```python
from build123d import *

# Parameters (mm, degrees)
BOSS_EXTRUDE1_DEPTH = 30
SKETCH2_W           = 20
SKETCH2_H           = 8
BOSS_EXTRUDE2_DEPTH = 30
BOSS_EXTRUDE3_DEPTH = 30
FILLET2_R           = 35
FILLET3_R           = 3
SKETCH5_R           = 2.778125
CUT_EXTRUDE2_DEPTH  = 9
SKETCH6_R           = 24.13
BOSS_EXTRUDE4_DEPTH = 30
FILLET4_R           = 40
FILLET5_R           = 10
FILLET6_R           = 2


with BuildPart() as part:
    # Sketch1 → Boss-Extrude1 (new body)
    with BuildSketch(Plane.XY):
        with BuildLine():
            ThreePointArc((66.675, 0), (0, 66.675), (-66.675, 0))
            Line((-66.675, 0), (-57.15, 0))
            ThreePointArc((-57.15, 0), (0, 57.15), (57.15, 0))
            Line((57.15, 0), (66.675, 0))
        make_face()
    extrude(amount=BOSS_EXTRUDE1_DEPTH)

    # Sketch2 → Boss-Extrude2 (add)
    with BuildSketch(Plane.XY.offset(30)):
        with Locations((-71.9125, 4)):
            Rectangle(SKETCH2_W, SKETCH2_H)
        with Locations((71.9125, 4)):
            Rectangle(SKETCH2_W, SKETCH2_H)
    extrude(amount=-BOSS_EXTRUDE2_DEPTH)

    # Sketch4 → Boss-Extrude3 (add)
    with BuildSketch(Plane.XY.offset(30)):
        with BuildLine():
            Line((-89.9125, 40), (-89.9125, 35))
            Line((-89.9125, 35), (-81.9125, 35))
            Line((-81.9125, 35), (-56.749939427, 35))
            ThreePointArc((-56.749939427, 35), (-55.103585117, 37.538653841), (-53.343749634, 40))
            Line((-53.343749634, 40), (-89.9125, 40))
        make_face()
        Polygon((-89.9125, 0), (-81.9125, 0), (-81.9125, 8), (-81.9125, 35), (-89.9125, 35), align=None)
        with BuildLine():
            Line((89.9125, 40), (53.343749634, 40))
            ThreePointArc((53.343749634, 40), (55.103585117, 37.538653841), (56.749939427, 35))
            Line((56.749939427, 35), (81.9125, 35))
            Line((81.9125, 35), (89.9125, 35))
            Line((89.9125, 35), (89.9125, 40))
        make_face()
        Polygon((89.9125, 0), (89.9125, 35), (81.9125, 35), (81.9125, 8), (81.9125, 0), align=None)
    extrude(amount=-BOSS_EXTRUDE3_DEPTH)

    # Fillet2
    fillet2_edges = [part.edges().sort_by_distance(p)[0] for p in [
        (-53.343749634, 40, 15),
        (53.343749634, 40, 15),
    ]]
    fillet(fillet2_edges, radius=FILLET2_R)

    # Fillet3
    fillet3_edges = [part.edges().sort_by_distance(p)[0] for p in [
        (-56.749939427, 35, 15),
        (56.749939427, 35, 15),
    ]]
    fillet(fillet3_edges, radius=FILLET3_R)

    # Sketch5 → Cut-Extrude2 (cut, through all)
    with BuildSketch(Plane(origin=(0, 8, 0), x_dir=(1, 0, 0), z_dir=(0, 1, 0))):
        with Locations((-74.052910047, -15)):
            Circle(SKETCH5_R)
        with Locations((74.052910047, -15)):
            Circle(SKETCH5_R)
    extrude(amount=-CUT_EXTRUDE2_DEPTH, mode=Mode.SUBTRACT)

    # Sketch6 → Boss-Extrude4 (add)
    with BuildSketch(Plane.XY.offset(30)):
        with BuildLine():
            Line((-98.9125, 44), (-118.9125, 44))
            ThreePointArc((-118.9125, 44), (-135.746949407, -15.213991129), (-90.279215199, 26.287582073))
            Line((-90.279215199, 26.287582073), (-79.281188547, 40))
            Line((-79.281188547, 40), (-98.9125, 44))
        make_face()
        with Locations((-118.9125, 12)):
            Circle(SKETCH6_R, mode=Mode.SUBTRACT)
        with BuildLine():
            Line((98.9125, 44), (79.281188547, 40))
            Line((79.281188547, 40), (90.279215199, 26.287582073))
            ThreePointArc((90.279215199, 26.287582073), (135.746949407, -15.213991129), (118.9125, 44))
            Line((118.9125, 44), (98.9125, 44))
        make_face()
        with Locations((118.9125, 12)):
            Circle(SKETCH6_R, mode=Mode.SUBTRACT)
    extrude(amount=-BOSS_EXTRUDE4_DEPTH)

    # Fillet4
    fillet4_edges = [part.edges().sort_by_distance(p)[0] for p in [
        (-98.9125, 44, 15),
        (-79.281188547, 40, 15),
        (79.281188547, 40, 15),
        (98.9125, 44, 15),
    ]]
    fillet(fillet4_edges, radius=FILLET4_R)

    # Fillet5
    fillet5_edges = [part.edges().sort_by_distance(p)[0] for p in [
        (-81.9125, 35, 15),
        (81.9125, 35, 15),
    ]]
    fillet(fillet5_edges, radius=FILLET5_R)

    # Fillet6
    fillet6_edges = [part.edges().sort_by_distance(p)[0] for p in [
        (-81.9125, 8, 15),
        (-66.193320093, 8, 15),
        (66.193320093, 8, 15),
        (81.9125, 8, 15),
    ]]
    fillet(fillet6_edges, radius=FILLET6_R)


solid = part.part
```
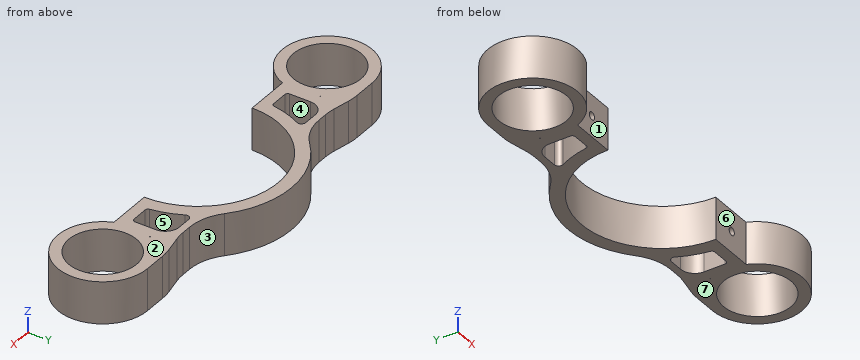
Build history of the part. All positions in model axes, mm. Face numbers are marked on the shaded views. A direction names the side the tool comes from. Round coordinates to 2 decimals unless told otherwise and drop trailing zeros. Write each loop counter-clockwise with the first axis right and the second up, starting at its lowest first coordinate (ties: lowest second). Pieces come first, ordered by that corner, then holes.
1) Pin check, flat tips, straight feed: pin 1 (1.5 mm diameter, centred on y = 25.5, z = 21.5, fed in from +X); pin 2 (3 mm diameter, centred on x = 35.5, z = 9.5, fed in from +Y); pin 3 (4 mm diameter, centred on y = -7, z = 26, fed in from -X). Stop position of each tip, or through.
2) Drill centre lines: probe 1 along X at (y, z) = (5.75, 15); probe 2 along X at (y, z) = (33.5, 4.75); probe 3 along Y at (x, z) = (120.5, 2.25). Where is each one in solid material? Low to high.
3) Mould opens along Y. For the marked faces 1, 2, 3 and 4 say: +Y half, -Y half, draft (parallel to the pull), parting line (faces both ways), or undercut.
4) Band-saw the part on B-B, the plane z = 9. Give the number of separate pieces and of enclosed holes in the cut face, and give its area (3 significant figures).
5) 3-axis set-ups, long thin cutter, end or side, ignore diameter. For the marked faces 5, 6 and 7: which of +Z, -Z, +X, -X, +Y, -Y reach the whole face in a straight line?
6) Band-saw the part on D-D, the plane x = -127. List the corners of the cut face in (y, z).
7) Band-saw the part on A-A, the plane x = 113.5. List the corners of the cut face in (y, z), and give its area (3 significant figures).
8) Band-saw the part on C-C, the plane x = 0. List the corners of the cut face in (y, z) (3 decimals).
Ans:
1. pin 1: stops at x = 148.26
1. pin 2: stops at y = 57.35
1. pin 3: stops at x = -146.02
2. probe 1: x = -150.3 to -142.22, -95.61 to -76.83, -71.27 to -56.86, 56.86 to 71.27, 76.83 to 95.61, 142.22 to 150.3
2. probe 2: x = -142.61 to -129.87, -107.96 to -77.18, -59.29 to -46.3, 46.3 to 59.29, 77.18 to 107.96, 129.87 to 142.61
2. probe 3: y = -19.96 to -12.08, 36.08 to 43.96
3. face 1: -Y half
3. face 2: draft
3. face 3: +Y half
3. face 4: undercut
4. separate pieces: 1
4. enclosed holes: 6
4. area: 6,100 mm2
5. face 5: +Z, -Z
5. face 6: +Z, -Z, -Y
5. face 7: -Z, +X, -X, +Y, -Y
6. outline: (-18.96, 0) - (-10.73, 0) - (-10.73, 30) - (-18.96, 30) - close; (34.73, 0) - (42.96, 0) - (42.96, 30) - (34.73, 30) - close
7. outline: (-19.54, 0) - (-11.52, 0) - (-11.52, 30) - (-19.54, 30) - close; (35.52, 0) - (44, 0) - (44, 30) - (35.52, 30) - close
7. area: 495 mm2
8. outline: (57.15, 0) - (66.675, 0) - (66.675, 30) - (57.15, 30) - close
